Here's the drawing with two shaded views (mm, measured from the low corner). I have some questions. Round coordinates to 2 decimals unless told otherwise and drop trailing zeros. Write each loop counter-clockwise with the first axis right and the second up, starting at its lowest first coordinate (ties: lowest second). Pieces come first, ordered by that corner, then holes. Notation, with made-up numbers: M -28.5,75.5 L -13.5,75.5 A26 cw -13.5,104.5 Z; hole C -19.75,-29 d7. An arc over 180 degrees is marked long. Write item = value, one per line. Start each with the question number.
(1) I want a section at A-A (y = 67.5). List the corners of the cut face in (x, z) for me, and give its area (3 significant figures).
(2) I want a section at C-C (y = 37.5). List the corners of the cut face in (x, z) for me, and give its area (3 significant figures).
(3) I want a section at D-D (z = 1.85). List the corners of the cut face in (x, y) for me, and give its area (3 significant figures).
(4) I need wall thicknesses on line 1 along Y through (x, z) = (37.5, 2.05); line 2 along X through (y, z) = (38, 2); line 3 along X through (y, z) = (43.5, 0.75). Which ranges of each line are inside material? Lowest first, please.
(5) Will this pin go through, and if not, where does the flat tip stop? pin 1 Ø1.5 at (x, z) = (63, 0.5) entering from +Y.
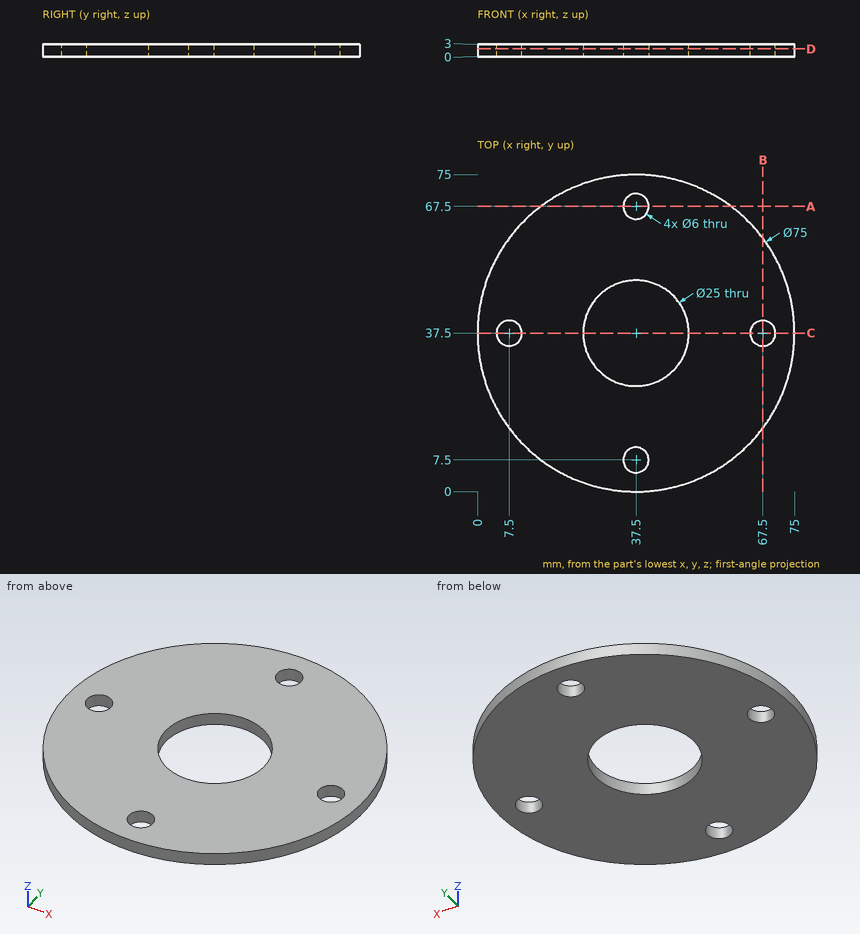
Returned:
q1.outline = M 15,0 L 34.5,0 L 34.5,3 L 15,3 Z; M 40.5,0 L 60,0 L 60,3 L 40.5,3 Z
q1.area = 117 mm²
q2.outline = M 0,0 L 4.5,0 L 4.5,3 L 0,3 Z; M 10.5,0 L 25,0 L 25,3 L 10.5,3 Z; M 50,0 L 64.5,0 L 64.5,3 L 50,3 Z; M 70.5,0 L 75,0 L 75,3 L 70.5,3 Z
q2.area = 114 mm²
q3.outline = C 37.5,37.5 d75; hole C 7.5,37.5 d6; hole C 37.5,37.5 d25; hole C 37.5,7.5 d6; hole C 37.5,67.5 d6; hole C 67.5,37.5 d6
q3.area = 3,810 mm²
q4.line_1 = 0 to 4.5, 10.5 to 25, 50 to 64.5, 70.5 to 75
q4.line_2 = 0 to 4.54, 10.46 to 25.01, 49.99 to 64.54, 70.46 to 75
q4.line_3 = 0.48 to 26.53, 48.47 to 74.52
q5.pin_1 = 65.67
